Design review of the part built by this model. Coordinates are the model's own, in mm. Face numbers are marked on the shaded views. Coordinates: 2 decimals unless noted, no trailing zeros. Order: outer loops, then holes, each group sorted by start corner. A loop starts at its lowest first (then second) coordinate and runs counter-clockwise, first axis right, second up. Notation, with made-up numbers: M -28,13 L 10,13 A32 cw 10,44 Z; hole C 86,50 d8. An arc over 180 degrees is marked long. Use CSV: the item, a comma, the result in double quotes.
```python
from build123d import *

# Parameters (mm, degrees)
FILLET1_R = 0.6
FILLET2_R = 1


with BuildPart() as part:
    # Sketch1 → Revolve1 (revolve)
    with BuildSketch(Plane.XY):
        Polygon((0, 16.080825938), (0, 19.563235604), (1.2, 19.999999886), (7, 19.999999886), (7, 17.398922974), (10, 16), (10, 15), (8.35338, 15.349999886), align=None)
    revolve(axis=Axis((0, 0, 0), (1, 0, 0)))

    # Fillet1
    fillet1_edges = [part.edges().sort_by_distance(p)[0] for p in [
        (0, -16.080825938, 0),
        (7, -17.398922974, 0),
    ]]
    fillet(fillet1_edges, radius=FILLET1_R)

    # Fillet2
    fillet2_edges = [part.edges().sort_by_distance(p)[0] for p in [
        (7, -19.999999886, 0),
    ]]
    fillet(fillet2_edges, radius=FILLET2_R)


solid = part.part
```
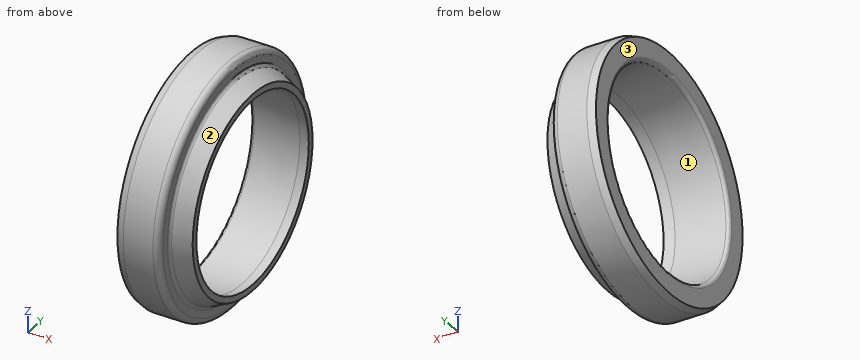
(1) Clearance check with flat-ended pins moving along their axes: P1, Ø1.5, axis at x = 4, y = 13.5, coming from the -Z side; P2, Ø6, axis at x = 2, z = -13.5, coming from the -Y side; P3, Ø1.5, axis at x = 7, z = -2.5, coming from the +Y side. State where each tip first meets the part, or that it passes through.
The answers:
P1,"stops at z = -15.41"
P2,"stops at y = -17.02"
P3,"stops at y = 19.83"
(2) Wall thickness on probe 1 along Y at (x, z) = (0.75, 12.5); probe 2 along Y at (x, z) = (7.25, 13); probe 3 along Z at (x, y) = (1, 13.5): over which ranges is each line inside the solid? List them lowest first.
The answers:
probe 1,"y = -15.4 to -10.01, 10.01 to 15.4"
probe 2,"y = -11.41 to -8.34, 8.34 to 11.41"
probe 3,"z = -14.66 to -8.58, 8.58 to 14.66"
(3) Add section C-C on x = 5.5. State the section outline as (y, z) points.
The answers:
outline,"C 0,0 d40; hole C 0,0 d31.2"
(4) Add section D-D on x = 9. State the section outline as (y, z) points.
The answers:
outline,"C 0,0 d32.93; hole C 0,0 d30.43"
(5) Add section A-A on z = 0. State the section outline as (x, y) points, and give its area (3 significant figures).
The answers:
outline,"M 0,-19.56 L 1.2,-20 L 6,-20 A1 ccw 7,-19 L 7,-17.78 A0.6 cw 7.35,-17.24 L 10,-16 L 10,-15 L 8.35,-15.35 L 0.55,-16.03 A0.6 ccw 0,-16.63 Z; M 0,16.63 A0.6 ccw 0.55,16.03 L 8.35,15.35 L 10,15 L 10,16 L 7.35,17.24 A0.6 cw 7,17.78 L 7,19 A1 ccw 6,20 L 1.2,20 L 0,19.56 Z"
area,"66.6 mm2"
(6) The part is to be moulded in two halves that separate along Y. For the marked faces 1, 2 and 3, say which applies: pulls with the +Y half, pulls with the -Y half, needs draft (parallel to the pull), parting line crosses it, or undercut.
The answers:
face 1,"undercut"
face 2,"parting line crosses it"
face 3,"needs draft"
